```python
from build123d import *

# Parameters (mm, degrees)
SKETCH_1_W          = 160
SKETCH_1_H          = 100
EXTRUDE_1_DEPTH     = 2
SKETCH_2_R          = 1.7
CUT_EXTRUDE_1_DEPTH = 95.361008897
SKETCH_3_W          = 135
SKETCH_3_H          = 70
EXTRUDE_2_DEPTH     = 22


with BuildPart() as part:
    # 스케치1 → 보스-돌출1 (new body)
    with BuildSketch(Plane(origin=(0, 0, 0), x_dir=(1, 0, 0), z_dir=(0, 1, 0))):
        Rectangle(SKETCH_1_W, SKETCH_1_H)
    extrude(amount=EXTRUDE_1_DEPTH)

    # 스케치2 → 컷-돌출1 (cut, through all)
    with BuildSketch(Plane(origin=(0, 2, 0), x_dir=(1, 0, 0), z_dir=(0, 1, 0))):
        with Locations(Location((77.3, 47.3, 0), (0, 0, 270))):
            Circle(SKETCH_2_R)
        with Locations(Location((77.3, -47.3, 0), (0, 0, 90))):
            Circle(SKETCH_2_R)
        with Locations(Location((-77.3, -47.3, 0), (0, 0, 270))):
            Circle(SKETCH_2_R)
        with Locations(Location((-77.3, 47.3, 0), (0, 0, 90))):
            Circle(SKETCH_2_R)
    extrude(amount=-CUT_EXTRUDE_1_DEPTH, mode=Mode.SUBTRACT)

    # 스케치3 → 보스-돌출2 (add)
    with BuildSketch(Plane(origin=(0, 2, 0), x_dir=(1, 0, 0), z_dir=(0, 1, 0))):
        Rectangle(SKETCH_3_W, SKETCH_3_H)
    extrude(amount=EXTRUDE_2_DEPTH)


solid = part.part
```
Check sheet for the modelled part. Datum: model origin and axes. Units: mm. A direction names the side the tool comes from. Round coordinates to 2 decimals unless told otherwise and drop trailing zeros. Order: outer loops, then holes, each group sorted by start corner. A loop starts at its lowest first (then second) coordinate and runs counter-clockwise, first axis right, second up.
1) Go/stop test with flat-tipped pins: pin 1 Ø1.5 at (y, z) = (8, -3.5) entering from +X; pin 2 Ø2.5 at (x, z) = (-77.3, -47.3) entering from +Y; pin 3 Ø6.5 at (x, y) = (-4, 8) entering from -Z; pin 4 Ø4 at (y, z) = (8, -12.5) entering from -X. Record where each tip stops, or that it passes through.
2) Mould release check, pull along X, two halves, no side actions. Record for faces 5 (the cylindrical face through (-78.733, 1.014, -48.214)), 6 (the flat face through (-1, 24, 0)), 7 (the flat face through (67.5, 13, 0)): +X half, -X half, draft (parallel to the pull), parting line (faces both ways), or undercut.
3) Section check D-D (z = -24). Record the boundary of the cut face in (x, y), and give its area (3 significant figures).
4) Section check C-C (x = -9). Record the boundary of the cut face in (y, z).
5) Section check A-A (z = -47.3). Record the boundary of the cut face in (x, y).
6) Section check B-B (x = 77.3). Record the boundary of the cut face in (y, z), and give its area (3 significant figures).
7) Tool access check on faces 1 (the cylindrical face through (-78.8, 1, 48.1)), 2 (the flat face through (-1, 13, 35)), 3 (the flat face through (-67.5, 13, 0)), 4 (the flat face through (-1, 13, -35)). Record the directions out of +Z, -Z, +X, -X, +Y, -Y that give a thin tool (end or side, any length) a straight path to the whole face; none if there is none.
8) Scan lines: line 1 (X direction, y = 1.55, z = -47.3); line 2 (Z direction, x = 77.3, y = 1.3); line 3 (Z direction, x = -29, y = 13). Record each from-to range of solid material in increasing order.
Result:
1. pin 1: stops at x = 67.5
1. pin 2: passes through
1. pin 3: stops at z = -35
1. pin 4: stops at x = -67.5
2. face 5: undercut
2. face 6: draft
2. face 7: +X half
3. outline: (-80, 0) - (80, 0) - (80, 2) - (67.5, 2) - (67.5, 24) - (-67.5, 24) - (-67.5, 2) - (-80, 2) - close
3. area: 3,290 mm2
4. outline: (0, -50) - (2, -50) - (2, -35) - (24, -35) - (24, 35) - (2, 35) - (2, 50) - (0, 50) - close
5. outline: (-80, 0) - (-79, 0) - (-79, 2) - (-80, 2) - close; (-75.6, 0) - (75.6, 0) - (75.6, 2) - (-75.6, 2) - close; (79, 0) - (80, 0) - (80, 2) - (79, 2) - close
6. outline: (0, -50) - (2, -50) - (2, -49) - (0, -49) - close; (0, -45.6) - (2, -45.6) - (2, 45.6) - (0, 45.6) - close; (0, 49) - (2, 49) - (2, 50) - (0, 50) - close
6. area: 186 mm2
7. face 1: +Y, -Y
7. face 2: +Z, +X, -X, +Y
7. face 3: +Z, -Z, -X, +Y
7. face 4: -Z, +X, -X, +Y
8. line 1: x = -80 to -79, -75.6 to 75.6, 79 to 80
8. line 2: z = -50 to -49, -45.6 to 45.6, 49 to 50
8. line 3: z = -35 to 35
